```python
from build123d import *

# Parameters (mm, degrees)
F0_W     = 2.97095
F0_H     = 0.218032
F0_W_2   = 1.209654
F0_H_2   = 0.189883
F1_DEPTH = 0.5


with BuildPart() as f1:
    # F0 (on Front) → F1 (new body)
    with BuildSketch(Plane.XZ):
        with BuildLine():
            ThreePointArc((-44.103578, 8.935158), (-43.980027, 8.789603), (-43.794962, 8.742675))
            Line((-43.794962, 8.742675), (-42.037207, -5.533148))
            Line((-42.037207, -5.533148), (-42.346001, -6.031972))
            ThreePointArc((-42.346001, -6.031972), (-42.678832, -6.130309), (-42.904774, -6.39374))
            Line((-42.904774, -6.39374), (-42.904774, -6.481908))
            ThreePointArc((-42.904774, -6.481908), (-42.780729, -6.63127), (-42.601286, -6.705408))
            ThreePointArc((-42.601286, -6.705408), (-40.726024, -7.06924), (-38.818597, -6.965784))
            Line((-38.818597, -6.965784), (-38.818597, -6.532135))
            Line((-38.818597, -6.532135), (-38.818597, -6.314103))
            Line((-38.818597, -6.314103), (-38.818597, -6.031972))
            Line((-38.818597, -6.031972), (-38.307915, -6.031972))
            Line((-38.307915, -6.031972), (-40.231944, -5.081834))
            Line((-40.231944, -5.081834), (-39.30556, 7.032427))
            ThreePointArc((-39.30556, 7.032427), (-37.733332, 7.518913), (-36.741034, 8.831892))
            ThreePointArc((-36.741034, 8.831892), (-36.774021, 8.995548), (-36.920728, 9.075224))
            Line((-36.920728, 9.075224), (-38.264113, 9.075224))
            Line((-38.264113, 9.075224), (-38.264113, 9.545864))
            Line((-38.264113, 9.545864), (-37.425197, 9.545864))
            Line((-37.425197, 9.545864), (-37.145558, 9.720638))
            Line((-37.145558, 9.720638), (-37.145558, 12.546355))
            Line((-37.145558, 12.546355), (-37.425197, 12.74232))
            Line((-37.425197, 12.74232), (-37.425197, 13.201373))
            Line((-37.425197, 13.201373), (-36.788988, 13.201373))
            Line((-36.788988, 13.201373), (-36.788988, 13.403278))
            ThreePointArc((-36.788988, 13.403278), (-37.723861, 14.44951), (-38.928528, 15.168793))
            ThreePointArc((-38.928528, 15.168793), (-38.9336, 15.170855), (-38.938675, 15.17291))
            Line((-38.938675, 15.17291), (-38.938675, 15.505459))
            Line((-38.938675, 15.505459), (-38.938675, 15.838007))
            ThreePointArc((-38.938675, 15.838007), (-37.566496, 15.944642), (-36.254536, 16.360583))
            Line((-36.254536, 16.360583), (-36.254536, 16.604704))
            Line((-36.254536, 16.604704), (-36.254536, 16.794587))
            Line((-36.254536, 16.794587), (-36.254536, 16.906913))
            Line((-36.254536, 16.906913), (-35.874481, 16.906913))
            Line((-35.874481, 16.906913), (-35.874481, 17.536379))
            ThreePointArc((-35.874481, 17.536379), (-37.632307, 18.162802), (-39.486278, 18.375282))
            Line((-39.486278, 18.375282), (-41.803283, 18.375282))
            Line((-41.803283, 18.375282), (-42.881891, 18.375282))
            ThreePointArc((-42.881891, 18.375282), (-43.559562, 18.134035), (-44.166764, 17.74836))
            Line((-44.166764, 17.74836), (-44.166764, 16.790975))
            ThreePointArc((-44.166764, 16.790975), (-43.554395, 16.437088), (-42.881891, 16.21807))
            Line((-42.881891, 16.21807), (-42.582278, 16.21807))
            Line((-42.582278, 16.21807), (-42.613738, 16.00273))
            Line((-42.613738, 16.00273), (-42.964101, 16.00273))
            Line((-42.964101, 16.00273), (-43.854554, 14.518307))
            Line((-43.854554, 14.518307), (-43.854554, 12.956257))
            Line((-43.854554, 12.956257), (-42.603236, 12.956257))
            Line((-42.603236, 12.956257), (-42.603236, 12.76462))
            Line((-42.603236, 12.76462), (-43.582644, 12.76462))
            Line((-43.582644, 12.76462), (-43.582644, 9.575224))
            Line((-43.582644, 9.575224), (-40.582644, 9.575224))
            Line((-40.582644, 9.575224), (-40.582644, 9.075224))
            Line((-40.582644, 9.075224), (-43.264113, 9.075224))
            Line((-43.264113, 9.075224), (-43.901596, 9.075224))
            ThreePointArc((-43.901596, 9.075224), (-44.030593, 9.045576), (-44.103578, 8.935158))
        make_face()
        with Locations((-37.333122, -6.423119)):
            Rectangle(F0_W, F0_H)
        Polygon((-35.847647, -6.314103), (-35.847647, -6.532135), (-35.847647, -6.597614), (-35.317635, -6.597614), (-35.317635, -6.240905), (-35.847647, -6.240905), align=None)
        with BuildLine():
            ThreePointArc((-38.938675, 15.17291), (-38.9336, 15.170855), (-38.928528, 15.168793))
            ThreePointArc((-38.928528, 15.168793), (-38.929196, 15.337259), (-38.938675, 15.505459))
            Line((-38.938675, 15.505459), (-38.938675, 15.17291))
        make_face()
        with Locations((-35.649709, 16.699645)):
            Rectangle(F0_W_2, F0_H_2)
        Polygon((-35.044882, 16.887183), (-35.044882, 16.794587), (-35.044882, 16.604704), (-35.044882, 16.541855), (-34.755295, 16.541855), (-34.755295, 16.887183), align=None)
    extrude(amount=F1_DEPTH)


solid = f1.part
```
The model under review builds one solid part; all positions refer to its coordinate system, in mm. A direction names the side the tool comes from. Give positions to 0.01 mm unless a question says otherwise; leave off trailing zeros. Write each loop counter-clockwise with the first axis right and the second up, starting at its lowest first coordinate (ties: lowest second). Pieces come first, ordered by that corner, then holes. Notation, with made-up numbers: M 12,88.25 L 24,88.25 A14 cw 24,106.25 Z; hole C 46,-28 d6. An arc over 180 degrees is marked long. Write item = value, one per line. Start each with the question number.
Q1. For line 1 (X direction, y = -0.1, z = 17); line 2 (Z direction, x = -41, y = -0.05); line 3 (Z direction, x = -35.25, y = -0.3), list the stretches that pass through material, from the lowest coordinate up.
Q2. Machinability: for faces 1 (the face through (-39.775, -0.246, 0.89)), 2 (the face through (-43.403, -0.246, 15.271)), 3 (the face through (-40.6, -0.5, 8.7)), which of the approach directions +Z, -Z, +X, -X, +Y, -Y give a long, thin tool a straight path to every point of the face, cutting with its end or side? Answer none if there is none.
Q3. We need section C-C (z = 2.5). State the section outline as (x, y) points, plus the area to 3 significant figures.
Q4. We need section B-B (z = 11.75). State the section outline as (x, y) points, plus the area to 3 significant figures.
Q5. Mouldability with a two-part tool opening along Z and no side actions: class faces 4 (the face through (-42.928, -0.246, 1.705)), 5 (the face through (-37.607, -0.246, 18.157)), 6 (the face through (-40.6, 0, 8.7)) as released by +Z, released by -Z, zero draft, split by the parting line, or undercut.
Q6. We need section A-A (x = -39.75). State the section outline as (y, z) points.
Result set:
q1.line_1 = -44.17 to -35.87
q1.line_2 = -7.05 to 9.08, 9.58 to 18.38
q1.line_3 = 16.6 to 16.79
q2.face_1 = +X, +Y, -Y
q2.face_2 = -X, +Y, -Y
q2.face_3 = +Z, -Z, +X, -X, -Y
q3.outline = M -43.03,-0.5 L -39.65,-0.5 L -39.65,0 L -43.03,0 Z
q3.area = 1.69 mm2
q4.outline = M -43.58,-0.5 L -37.15,-0.5 L -37.15,0 L -43.58,0 Z
q4.area = 3.22 mm2
q5.face_4 = undercut
q5.face_5 = released by +Z
q5.face_6 = zero draft
q6.outline = M -0.5,-7.08 L 0,-7.08 L 0,-5.32 L -0.5,-5.32 Z; M -0.5,1.22 L 0,1.22 L 0,18.38 L -0.5,18.38 Z
